Read the model definition and answer for the solid it produces. Units are mm, in the model's axes. A direction names the side the tool comes from. Round coordinates to 2 decimals unless told otherwise and drop trailing zeros. Order: outer loops, then holes, each group sorted by start corner. A loop starts at its lowest first (then second) coordinate and runs counter-clockwise, first axis right, second up. Notation, with made-up numbers: M 29,-5.5 L 76,-5.5 A12 cw 76,15.5 Z; hole C 22.5,56 d1. An arc over 180 degrees is marked long. Answer as CSV lines item,"result".
```python
from build123d import *

# Parameters (mm, degrees)
SKETCH1_R             = 0.3
BOSS_EXTRUDE1_DEPTH   = 4.72
BOSS_EXTRUDE1_2_DEPTH = 4.72


with BuildPart() as part:
    # Sketch1 → Boss-Extrude1 (new body)
    with BuildSketch(Plane(origin=(0, 0, 0), x_dir=(1, 0, 0), z_dir=(0, 1, 0))):
        with Locations(Location((-2.5, 0, 0), (0, 0, 270))):
            Circle(SKETCH1_R)
    extrude(amount=-BOSS_EXTRUDE1_DEPTH)



with BuildPart() as body_2:
    # Sketch1 → Boss-Extrude1 2 (new body)
    with BuildSketch(Plane(origin=(0, 0, 0), x_dir=(1, 0, 0), z_dir=(0, 1, 0))):
        with Locations(Location((2.5, 0, 0), (0, 0, 90))):
            Circle(SKETCH1_R)
    extrude(amount=-BOSS_EXTRUDE1_2_DEPTH)


with BuildPart() as part_1:
    add(part.part)

    add(body_2.part)  # Revolve1 merges body 2
    # Sketch3 → Revolve1 (revolve)
    with BuildSketch(Plane.XY):
        with BuildLine():
            Line((5, 0.4), (5, 0.650521697))
            ThreePointArc((5, 0.650521697), (4.937148311, 0.893217708), (4.764394584, 1.074898303))
            ThreePointArc((4.764394584, 1.074898303), (4.528386612, 1.5), (4.764394584, 1.925101697))
            ThreePointArc((4.764394584, 1.925101697), (4.937148311, 2.106782292), (5, 2.349478303))
            Line((5, 2.349478303), (5, 19.6))
            ThreePointArc((5, 19.6), (4.853553391, 19.953553391), (4.5, 20.1))
            Line((4.5, 20.1), (4, 20.1))
            Line((4, 20.1), (4, 20))
            Line((4, 20), (0, 20))
            Line((0, 20), (0, 0))
            Line((0, 0), (4, 0))
            Line((4, 0), (4, -0.1))
            Line((4, -0.1), (4.5, -0.1))
            ThreePointArc((4.5, -0.1), (4.853553391, 0.046446609), (5, 0.4))
        make_face()
    revolve(axis=Axis((0, 0, 0), (0, 1, 0)))


solid = part_1.part
```
Item 1: A tool of negligible diameter and unlimited length cuts with its end or side. For faces 1 (the face through (-3, 20.1, 3)), 2 (the face through (0, 0, 0)), from which of +Z, -Z, +X, -X, +Y, -Y can it reach the whole face along a straight path? Write none if from no direction.
Ans:
face 1,"+Z, -Z, +X, -X, +Y"
face 2,"-Y"
Item 2: Flat-ended cylindrical pins translate along their axes: pin 1 (6 mm diameter, centred on x = 1.5, y = 14, fed in from +Z); pin 2 (1.5 mm diameter, centred on y = 12, z = -3.5, fed in from -X); pin 3 (2.5 mm diameter, centred on x = -1.5, z = 0.5, fed in from +Y); pin 4 (4 mm diameter, centred on x = 0, z = 0.5, fed in from -Y). Find the tip coordinate at first contact, or state that the pin passes through.
Ans:
pin 1,"z = 5"
pin 2,"x = -4.18"
pin 3,"y = 20"
pin 4,"y = 0"
Item 3: Determine the mould class of faces 3 (the face through (3, -0.1, 3)), 4 (the face through (-1.08, 11.1, 4.88)), 5 (the face through (0, 20, 0)) for opening direction Z: +Z half, -Z half, draft (parallel to the pull), parting line (faces both ways), or undercut.
Ans:
face 3,"draft"
face 4,"parting line"
face 5,"undercut"
Item 4: Find the intervals of material crossed by probe 1 along Y at (x, z) = (0.25, -3.5); probe 2 along Z at (x, y) = (2.5, -1.75); probe 3 along Z at (x, y) = (1.5, 2.75), in increasing order. Write a range as [from, to].
Ans:
probe 1,"[0, 20]"
probe 2,"[-0.3, 0.3]"
probe 3,"[-4.77, 4.77]"
Item 5: A cutting plane is placed at C-C, the plane y = 5.75. Determine the outline of the cut face in (x, z).
Ans:
outline,"C 0,0 d10"
Item 6: A cutting plane is placed at A-A, the plane x = 0. Determine the outline of the cut face in (y, z).
Ans:
outline,"M -0.1,-4.5 A0.5 ccw 0.4,-5 L 0.65,-5 A0.5 ccw 1.07,-4.76 A0.5 cw 1.93,-4.76 A0.5 ccw 2.35,-5 L 19.6,-5 A0.5 ccw 20.1,-4.5 L 20.1,-4 L 20,-4 L 20,4 L 20.1,4 L 20.1,4.5 A0.5 ccw 19.6,5 L 2.35,5 A0.5 ccw 1.93,4.76 A0.5 cw 1.07,4.76 A0.5 ccw 0.65,5 L 0.4,5 A0.5 ccw -0.1,4.5 L -0.1,4 L 0,4 L 0,-4 L -0.1,-4 Z"
